from build123d import *

# Parameters (mm, degrees)
F0_R     = 2.54
F0_R_2   = 1.4986
F0_R_3   = 6.360074
F0_R_4   = 1.5875
F1_DEPTH = 19.05


with BuildPart() as f1:
    # F0 (on Top) → F1 (new body)
    with BuildSketch(Plane.XY):
        with BuildLine():
            Line((74.589707, 26.132662), (74.589707, 90.005893))
            ThreePointArc((74.589707, 90.005893), (0, 104.142881), (-74.589707, 90.005893))
            Line((-74.589707, 90.005893), (-74.589707, 26.132662))
            Line((-74.589707, 26.132662), (-45.310471, 26.132662))
            Line((-45.310471, 26.132662), (-45.310471, -26.132662))
            Line((-45.310471, -26.132662), (-74.589707, -26.132662))
            Line((-74.589707, -26.132662), (-74.589707, -90.005893))
            ThreePointArc((-74.589707, -90.005893), (0, -104.142881), (74.589707, -90.005893))
            Line((74.589707, -90.005893), (74.589707, -26.132662))
            Line((74.589707, -26.132662), (45.310471, -26.132662))
            Line((45.310471, -26.132662), (45.310471, 26.132662))
            Line((45.310471, 26.132662), (74.589707, 26.132662))
        make_face()
        with Locations((-67.364627, -86.673815)):
            Circle(F0_R, mode=Mode.SUBTRACT)
        with Locations((-44.504627, -86.673815)):
            Circle(F0_R, mode=Mode.SUBTRACT)
        with Locations((-19.447715, -77.214572)):
            Circle(F0_R_2, mode=Mode.SUBTRACT)
        with Locations((-31.509046, -60.463414)):
            Circle(F0_R_3, mode=Mode.SUBTRACT)
        with Locations((-67.364627, -43.681448)):
            Circle(F0_R, mode=Mode.SUBTRACT)
        with Locations((-67.364627, -35.219034)):
            Circle(F0_R, mode=Mode.SUBTRACT)
        with Locations((-44.504627, -43.681448)):
            Circle(F0_R, mode=Mode.SUBTRACT)
        with Locations((-44.504627, -35.219034)):
            Circle(F0_R, mode=Mode.SUBTRACT)
        with Locations((-19.447715, -40.127574)):
            Circle(F0_R_2, mode=Mode.SUBTRACT)
        with Locations((-31.293867, -12.662212)):
            Circle(F0_R_4, mode=Mode.SUBTRACT)
        with Locations((17.985267, -77.214572)):
            Circle(F0_R_2, mode=Mode.SUBTRACT)
        with Locations((31.674664, -59.26675)):
            Circle(F0_R_3, mode=Mode.SUBTRACT)
        with Locations((44.504627, -86.673815)):
            Circle(F0_R, mode=Mode.SUBTRACT)
        with Locations((67.364627, -86.673815)):
            Circle(F0_R, mode=Mode.SUBTRACT)
        with Locations((17.985267, -40.127574)):
            Circle(F0_R_2, mode=Mode.SUBTRACT)
        with Locations((19.506133, -27.889512)):
            Circle(F0_R_4, mode=Mode.SUBTRACT)
        with Locations((44.504627, -43.681448)):
            Circle(F0_R, mode=Mode.SUBTRACT)
        with Locations((44.504627, -35.219034)):
            Circle(F0_R, mode=Mode.SUBTRACT)
        with Locations((67.364627, -43.681448)):
            Circle(F0_R, mode=Mode.SUBTRACT)
        with Locations((67.364627, -35.219034)):
            Circle(F0_R, mode=Mode.SUBTRACT)
        with Locations((-67.364627, 35.219034)):
            Circle(F0_R, mode=Mode.SUBTRACT)
        with Locations((-67.364627, 43.681448)):
            Circle(F0_R, mode=Mode.SUBTRACT)
        with Locations((-44.504627, 35.219034)):
            Circle(F0_R, mode=Mode.SUBTRACT)
        with Locations((-44.504627, 43.681448)):
            Circle(F0_R, mode=Mode.SUBTRACT)
        with Locations((-31.281167, 15.293622)):
            Circle(F0_R_4, mode=Mode.SUBTRACT)
        with Locations((-19.447715, 40.127574)):
            Circle(F0_R_2, mode=Mode.SUBTRACT)
        with Locations((-67.364627, 86.673815)):
            Circle(F0_R, mode=Mode.SUBTRACT)
        with Locations((-44.504627, 86.673815)):
            Circle(F0_R, mode=Mode.SUBTRACT)
        with Locations((-30.464375, 64.66724)):
            Circle(F0_R_3, mode=Mode.SUBTRACT)
        with Locations((-19.447715, 77.214572)):
            Circle(F0_R_2, mode=Mode.SUBTRACT)
        with Locations((20.776133, 20.411722)):
            Circle(F0_R_4, mode=Mode.SUBTRACT)
        with Locations((17.985267, 40.127574)):
            Circle(F0_R_2, mode=Mode.SUBTRACT)
        with Locations((44.504627, 35.219034)):
            Circle(F0_R, mode=Mode.SUBTRACT)
        with Locations((44.504627, 43.681448)):
            Circle(F0_R, mode=Mode.SUBTRACT)
        with Locations((67.364627, 35.219034)):
            Circle(F0_R, mode=Mode.SUBTRACT)
        with Locations((67.364627, 43.681448)):
            Circle(F0_R, mode=Mode.SUBTRACT)
        with Locations((17.985267, 77.214572)):
            Circle(F0_R_2, mode=Mode.SUBTRACT)
        with Locations((32.647382, 62.834114)):
            Circle(F0_R_3, mode=Mode.SUBTRACT)
        with Locations((44.504627, 86.673815)):
            Circle(F0_R, mode=Mode.SUBTRACT)
        with Locations((67.364627, 86.673815)):
            Circle(F0_R, mode=Mode.SUBTRACT)
    extrude(amount=F1_DEPTH)


solid = f1.part
Verification items for the finished model (mm, model axes). A direction names the side the tool comes from. Give positions to 0.01 mm unless a question says otherwise; leave off trailing zeros. Write each loop counter-clockwise with the first axis right and the second up, starting at its lowest first coordinate (ties: lowest second). Pieces come first, ordered by that corner, then holes.
(1) Gauge pin test, flat ends, axial feed: pin 1 (2.5 mm diameter, centred on x = 17.99, y = 40.13, fed in from -Z); pin 2 (5.5 mm diameter, centred on y = 1.5, z = 11, fed in from -X); pin 3 (5 mm diameter, centred on y = -21, z = 16.5, fed in from +X). Record the tip position at first contact, or that the pin passes through.
(2) Material ranges on line 1 (Y direction, x = -31.5, z = 18); line 2 (Y direction, x = -64, z = 5.5); line 3 (X direction, y = 25, z = 1.25), recorded low to high.
(3) Access from +Z, -Z, +X, -X, +Y, -Y to the whole of each face (thin tool, end or side, straight path). Record for faces 1 (the face through (43.95, -46.16, 9.39)), 2 (the face through (-45.31, 0, 9)), 3 (the face through (45.31, 0, 9)).
(4) Cross-section at B-B (y = -19). Enter the section's corners in (x, z).
(5) Mould release check, pull along X, two halves, no side actions. Record for faces 4 (the face through (-67.92, 32.74, 9.39)), 5 (the face through (1.07, 104.14, 9.39)), 6 (the face through (-74.59, -58, 9)): +X half, -X half, draft (parallel to the pull), parting line (faces both ways), or undercut.
(6) Cross-section at C-C (z = 9.75). State how many separate pieces and enclosed holes the cut face has, plus the area to 3 significant figures.
(7) Cross-section at A-A (x = -57.5). Enter the section's corners in (y, z).
Worked out:
1. pin 1: passes through
1. pin 2: stops at x = -45.31
1. pin 3: stops at x = 45.31
2. line 1: y = -101.69 to -66.82, -54.1 to -14.24, -11.09 to 13.72, 16.87 to 58.39, 70.94 to 101.69
2. line 2: y = -93.84 to -26.13, 26.13 to 93.84
2. line 3: x = -45.31 to 45.31
3. face 1: +Z, -Z
3. face 2: +Z, -Z, -X
3. face 3: +Z, -Z, +X
4. outline: (-45.31, 0) - (45.31, 0) - (45.31, 19.05) - (-45.31, 19.05) - close
5. face 4: undercut
5. face 5: parting line
5. face 6: -X half
6. separate pieces: 1
6. enclosed holes: 40
6. area: 25,500 mm2
7. outline: (-95.87, 0) - (-26.13, 0) - (-26.13, 19.05) - (-95.87, 19.05) - close; (26.13, 0) - (95.87, 0) - (95.87, 19.05) - (26.13, 19.05) - close
